Build history of the part. All positions in model axes, mm. Face numbers are marked on the shaded views. Coordinates: 2 decimals unless noted, no trailing zeros. Order: outer loops, then holes, each group sorted by start corner. A loop starts at its lowest first (then second) coordinate and runs counter-clockwise, first axis right, second up. Notation, with made-up numbers: (16.25, 46.5) - (27.25, 46.5) arc R37 cw to (27.25, 83.5) - close; hole circle Ø10 at (61, -21). An arc over 180 degrees is marked (long way). One line per item, written item: value.
from build123d import *

# Parameters (mm, degrees)
BOSS_EXTRUDE1_DEPTH = 3.175
CUT_EXTRUDE1_REACH  = 154.646
SKETCH2_R           = 1.5875


with BuildPart() as part:
    # Sketch1 → Boss-Extrude1 (new body)
    with BuildSketch(Plane.XY):
        Polygon((0, 0), (25.4, 0), (132.228460039, -76.2), (0, -76.2), align=None)
    extrude(amount=BOSS_EXTRUDE1_DEPTH)

    # Sketch2 → Cut-Extrude1 (cut, up to next)
    with BuildSketch(Plane.XY.offset(3.175), mode=Mode.PRIVATE) as cut_extrude1_sk1:
        with Locations((12.7, -6.35)):
            Circle(SKETCH2_R)
    cut_extrude1_tool1 = extrude(cut_extrude1_sk1.sketch, amount=-CUT_EXTRUDE1_REACH, mode=Mode.PRIVATE) & part.part
    # Sketch2 → Cut-Extrude1 (cut, up to next)
    with BuildSketch(Plane.XY.offset(3.175), mode=Mode.PRIVATE) as cut_extrude1_sk2:
        with Locations((12.7, -25.4)):
            Circle(SKETCH2_R)
    cut_extrude1_tool2 = extrude(cut_extrude1_sk2.sketch, amount=-CUT_EXTRUDE1_REACH, mode=Mode.PRIVATE) & part.part
    # Sketch2 → Cut-Extrude1 (cut, up to next)
    with BuildSketch(Plane.XY.offset(3.175), mode=Mode.PRIVATE) as cut_extrude1_sk3:
        with Locations((12.7, -44.45)):
            Circle(SKETCH2_R)
    cut_extrude1_tool3 = extrude(cut_extrude1_sk3.sketch, amount=-CUT_EXTRUDE1_REACH, mode=Mode.PRIVATE) & part.part
    # Sketch2 → Cut-Extrude1 (cut, up to next)
    with BuildSketch(Plane.XY.offset(3.175), mode=Mode.PRIVATE) as cut_extrude1_sk4:
        with Locations((12.7, -63.5)):
            Circle(SKETCH2_R)
    cut_extrude1_tool4 = extrude(cut_extrude1_sk4.sketch, amount=-CUT_EXTRUDE1_REACH, mode=Mode.PRIVATE) & part.part
    # Sketch2 → Cut-Extrude1 (cut, up to next)
    with BuildSketch(Plane.XY.offset(3.175), mode=Mode.PRIVATE) as cut_extrude1_sk5:
        with Locations((35.739267083, -22.974679309)):
            Circle(SKETCH2_R)
    cut_extrude1_tool5 = extrude(cut_extrude1_sk5.sketch, amount=-CUT_EXTRUDE1_REACH, mode=Mode.PRIVATE) & part.part
    # Sketch2 → Cut-Extrude1 (cut, up to next)
    with BuildSketch(Plane.XY.offset(3.175), mode=Mode.PRIVATE) as cut_extrude1_sk6:
        with Locations((51.248167708, -34.037070616)):
            Circle(SKETCH2_R)
    cut_extrude1_tool6 = extrude(cut_extrude1_sk6.sketch, amount=-CUT_EXTRUDE1_REACH, mode=Mode.PRIVATE) & part.part
    # Sketch2 → Cut-Extrude1 (cut, up to next)
    with BuildSketch(Plane.XY.offset(3.175), mode=Mode.PRIVATE) as cut_extrude1_sk7:
        with Locations((66.757068333, -45.099461922)):
            Circle(SKETCH2_R)
    cut_extrude1_tool7 = extrude(cut_extrude1_sk7.sketch, amount=-CUT_EXTRUDE1_REACH, mode=Mode.PRIVATE) & part.part
    # Sketch2 → Cut-Extrude1 (cut, up to next)
    with BuildSketch(Plane.XY.offset(3.175), mode=Mode.PRIVATE) as cut_extrude1_sk8:
        with Locations((82.265968957, -56.161853228)):
            Circle(SKETCH2_R)
    cut_extrude1_tool8 = extrude(cut_extrude1_sk8.sketch, amount=-CUT_EXTRUDE1_REACH, mode=Mode.PRIVATE) & part.part
    # Sketch2 → Cut-Extrude1 (cut, up to next)
    with BuildSketch(Plane.XY.offset(3.175), mode=Mode.PRIVATE) as cut_extrude1_sk9:
        with Locations((97.774869582, -67.224244535)):
            Circle(SKETCH2_R)
    cut_extrude1_tool9 = extrude(cut_extrude1_sk9.sketch, amount=-CUT_EXTRUDE1_REACH, mode=Mode.PRIVATE) & part.part
    # Sketch2 → Cut-Extrude1 (cut, up to next)
    with BuildSketch(Plane.XY.offset(3.175), mode=Mode.PRIVATE) as cut_extrude1_sk10:
        with Locations((35.739267083, -38.574431081)):
            Circle(SKETCH2_R)
    cut_extrude1_tool10 = extrude(cut_extrude1_sk10.sketch, amount=-CUT_EXTRUDE1_REACH, mode=Mode.PRIVATE) & part.part
    # Sketch2 → Cut-Extrude1 (cut, up to next)
    with BuildSketch(Plane.XY.offset(3.175), mode=Mode.PRIVATE) as cut_extrude1_sk11:
        with Locations((51.248167708, -49.636822388)):
            Circle(SKETCH2_R)
    cut_extrude1_tool11 = extrude(cut_extrude1_sk11.sketch, amount=-CUT_EXTRUDE1_REACH, mode=Mode.PRIVATE) & part.part
    # Sketch2 → Cut-Extrude1 (cut, up to next)
    with BuildSketch(Plane.XY.offset(3.175), mode=Mode.PRIVATE) as cut_extrude1_sk12:
        with Locations((66.757068333, -60.699213694)):
            Circle(SKETCH2_R)
    cut_extrude1_tool12 = extrude(cut_extrude1_sk12.sketch, amount=-CUT_EXTRUDE1_REACH, mode=Mode.PRIVATE) & part.part
    # Sketch2 → Cut-Extrude1 (cut, up to next)
    with BuildSketch(Plane.XY.offset(3.175), mode=Mode.PRIVATE) as cut_extrude1_sk13:
        with Locations((82.265968957, -71.761605)):
            Circle(SKETCH2_R)
    cut_extrude1_tool13 = extrude(cut_extrude1_sk13.sketch, amount=-CUT_EXTRUDE1_REACH, mode=Mode.PRIVATE) & part.part
    add(cut_extrude1_tool1.solids().sort_by_distance((12.7, -6.35, 3.175))[0], mode=Mode.SUBTRACT)
    add(cut_extrude1_tool2.solids().sort_by_distance((12.7, -25.4, 3.175))[0], mode=Mode.SUBTRACT)
    add(cut_extrude1_tool3.solids().sort_by_distance((12.7, -44.45, 3.175))[0], mode=Mode.SUBTRACT)
    add(cut_extrude1_tool4.solids().sort_by_distance((12.7, -63.5, 3.175))[0], mode=Mode.SUBTRACT)
    add(cut_extrude1_tool5.solids().sort_by_distance((35.739267, -22.974679, 3.175))[0], mode=Mode.SUBTRACT)
    add(cut_extrude1_tool6.solids().sort_by_distance((51.248168, -34.037071, 3.175))[0], mode=Mode.SUBTRACT)
    add(cut_extrude1_tool7.solids().sort_by_distance((66.757068, -45.099462, 3.175))[0], mode=Mode.SUBTRACT)
    add(cut_extrude1_tool8.solids().sort_by_distance((82.265969, -56.161853, 3.175))[0], mode=Mode.SUBTRACT)
    add(cut_extrude1_tool9.solids().sort_by_distance((97.77487, -67.224245, 3.175))[0], mode=Mode.SUBTRACT)
    add(cut_extrude1_tool10.solids().sort_by_distance((35.739267, -38.574431, 3.175))[0], mode=Mode.SUBTRACT)
    add(cut_extrude1_tool11.solids().sort_by_distance((51.248168, -49.636822, 3.175))[0], mode=Mode.SUBTRACT)
    add(cut_extrude1_tool12.solids().sort_by_distance((66.757068, -60.699214, 3.175))[0], mode=Mode.SUBTRACT)
    add(cut_extrude1_tool13.solids().sort_by_distance((82.265969, -71.761605, 3.175))[0], mode=Mode.SUBTRACT)


solid = part.part
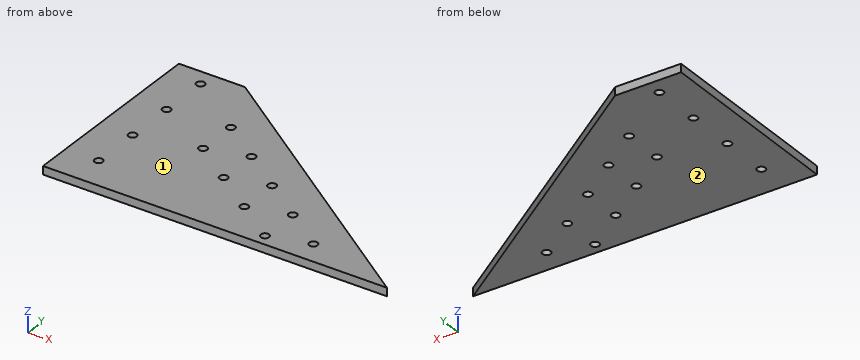
1. Band-saw the part on C-C, the plane z = 1.3. Count the separate pieces of the cut face and the enclosed holes in it, and give its area (3 significant figures).
Values found:
separate pieces: 1
enclosed holes: 13
area: 5,900 mm2
2. Band-saw the part on A-A, the plane x = 12.7. Give the cut face in (y, z) (1 decimal).
Values found:
outline: (-76.2, 0) - (-65.1, 0) - (-65.1, 3.2) - (-76.2, 3.2) - close; (-61.9, 0) - (-46, 0) - (-46, 3.2) - (-61.9, 3.2) - close; (-42.9, 0) - (-27, 0) - (-27, 3.2) - (-42.9, 3.2) - close; (-23.8, 0) - (-7.9, 0) - (-7.9, 3.2) - (-23.8, 3.2) - close; (-4.8, 0) - (0, 0) - (0, 3.2) - (-4.8, 3.2) - close
3. Band-saw the part on D-D, the plane x = 78. Give the cut face in (y, z) (3 decimals).
Values found:
outline: (-76.2, 0) - (-37.519, 0) - (-37.519, 3.175) - (-76.2, 3.175) - close
4. Probe line 1 along Y through (x, z) = (36, 2.4); line 2 along Y through (x, z) = (51, 2.4); line 3 along X through (y, z) = (-57, 2.2). List the from-to ranges inside material, lowest first.
Values found:
line 1: y = -76.2 to -40.14, -37.01 to -24.54, -21.41 to -7.56
line 2: y = -76.2 to -51.2, -48.07 to -35.61, -32.47 to -18.26
line 3: x = 0 to 80.92, 83.61 to 105.31
5. Two-plate mould, pull along Z, no slides. Class the marked faces 1 and 2: pulls with the +Z half, pulls with the -Z half, needs draft (parallel to the pull), parting line crosses it, or undercut.
Values found:
face 1: pulls with the +Z half
face 2: pulls with the -Z half
6. Band-saw the part on B-B, the plane y = -6.35. Give the cut face in (x, z) (1 decimal).
Values found:
outline: (0, 0) - (11.1, 0) - (11.1, 3.2) - (0, 3.2) - close; (14.3, 0) - (34.3, 0) - (34.3, 3.2) - (14.3, 3.2) - close
